CAD build for the part. Positions are in the model's coordinates, mm. A direction names the side the tool comes from. Give positions to 0.01 mm unless a question says otherwise; leave off trailing zeros. Write each loop counter-clockwise with the first axis right and the second up, starting at its lowest first coordinate (ties: lowest second). Pieces come first, ordered by that corner, then holes. Notation, with made-up numbers: (-9.5, 34.25) - (16.5, 34.25) arc R27 ccw to (16.5, 73.25) - close; hole circle Ø6 at (27, -2). An arc over 180 degrees is marked (long way). Answer as a JSON object with one key per item and string values.
from build123d import *

# Parameters (mm, degrees)
SKETCH_W     = 44.02
SKETCH_H     = 23
SKETCH_R     = 1
PAD_DEPTH    = 14.2
SKETCH001_R  = 3
PAD001_DEPTH = 3.36


with BuildPart() as part:
    # Sketch → Pad (new body, symmetric)
    with BuildSketch(Plane.YZ):
        Rectangle(SKETCH_W, SKETCH_H)
        with Locations((-20.1, -9.1)):
            Circle(SKETCH_R, mode=Mode.SUBTRACT)
        with Locations((20.1, -9.1)):
            Circle(SKETCH_R, mode=Mode.SUBTRACT)
        with Locations((-20.1, 9.1)):
            Circle(SKETCH_R, mode=Mode.SUBTRACT)
        with Locations((20.1, 9.1)):
            Circle(SKETCH_R, mode=Mode.SUBTRACT)
    extrude(amount=PAD_DEPTH, both=True)

    # Sketch001 (on Face10 of Pad) → Pad001 (join)
    with BuildSketch(Plane.YZ.offset(14.2)):
        with Locations((11.35, 0)):
            Circle(SKETCH001_R)
    pad001 = extrude(amount=PAD001_DEPTH)

    # Mirrored: Pad001 across YZ
    add(pad001.mirror(Plane.YZ))


solid = part.part
(1) Flat gauge pins, fed straight in: P1, Ø6, axis at y = -13, z = -8, coming from the +X side; P2, Ø1, axis at y = 0, z = -7, coming from the -X side; P3, Ø1.8, axis at y = 20.1, z = 9.1, coming from the +X side. Where does each tip first touch, or does it go through?
Answer key:
{"P1": "stops at x = 14.2", "P2": "stops at x = -14.2", "P3": "passes through"}
(2) Pull direction Z, two halves, no side cores. Call faces 4 (the face through (-0.199, -19.176, -9.483)), 5 (the face through (0, 0, -11.5)), 6 (the face through (0, -22.01, 0)): pulls with the +Z half, pulls with the -Z half, needs draft (parallel to the pull), parting line crosses it, or undercut.
Answer key:
{"face 4": "undercut", "face 5": "pulls with the -Z half", "face 6": "needs draft"}
(3) 3-axis set-ups, long thin cutter, end or side, ignore diameter. For faces 1 (the face through (17.56, 11, 0)), 2 (the face through (15.856, 8.353, 0.132)), 3 (the face through (-15.856, 8.353, 0.132)): which of +Z, -Z, +X, -X, +Y, -Y reach the whole face in a straight line?
Answer key:
{"face 1": "+Z, -Z, +X, +Y, -Y", "face 2": "+X", "face 3": "-X"}
(4) Saw through at D-D, the plane z = 0. Give the cut face in (x, y).
Answer key:
{"outline": "(-17.56, 8.35) - (-14.2, 8.35) - (-14.2, -22.01) - (14.2, -22.01) - (14.2, 8.35) - (17.56, 8.35) - (17.56, 14.35) - (14.2, 14.35) - (14.2, 22.01) - (-14.2, 22.01) - (-14.2, 14.35) - (-17.56, 14.35) - close"}
(5) Saw through at B-B, the plane y = 20.1. Give the cut face in (x, z), and give its area (3 significant figures).
Answer key:
{"outline": "(-14.2, -11.5) - (14.2, -11.5) - (14.2, -10.1) - (-14.2, -10.1) - close; (-14.2, -8.1) - (14.2, -8.1) - (14.2, 8.1) - (-14.2, 8.1) - close; (-14.2, 10.1) - (14.2, 10.1) - (14.2, 11.5) - (-14.2, 11.5) - close", "area": "540 mm²"}
(6) Probe L1, parallel to Z at x = 0.5, y = -20.1; L2, parallel to X at y = -17, z = 5.75. List the from-to ranges inside material, lowest first. Write a range as [from, to].
Answer key:
{"L1": "z = [-11.5, -10.1], [-8.1, 8.1], [10.1, 11.5]", "L2": "x = [-14.2, 14.2]"}
(7) Saw through at C-C, the plane y = 11. Give the cut face in (x, z), and give its area (3 significant figures).
Answer key:
{"outline": "(-17.56, -2.98) - (-14.2, -2.98) - (-14.2, -11.5) - (14.2, -11.5) - (14.2, -2.98) - (17.56, -2.98) - (17.56, 2.98) - (14.2, 2.98) - (14.2, 11.5) - (-14.2, 11.5) - (-14.2, 2.98) - (-17.56, 2.98) - close", "area": "693 mm²"}
(8) Saw through at A-A, the plane z = -9.1. Give the cut face in (x, y), and give its area (3 significant figures).
Answer key:
{"outline": "(-14.2, -22.01) - (14.2, -22.01) - (14.2, -21.1) - (-14.2, -21.1) - close; (-14.2, -19.1) - (14.2, -19.1) - (14.2, 19.1) - (-14.2, 19.1) - close; (-14.2, 21.1) - (14.2, 21.1) - (14.2, 22.01) - (-14.2, 22.01) - close", "area": "1,140 mm²"}
